Geometry check sheet. Reference: the model listing, model coordinates, mm. A direction names the side the tool comes from. Give positions to 0.01 mm unless a question says otherwise; leave off trailing zeros. Order: outer loops, then holes, each group sorted by start corner. A loop starts at its lowest first (then second) coordinate and runs counter-clockwise, first axis right, second up. Notation, with made-up numbers: M 63.5,36.25 L 81.5,36.25 A17 ccw 81.5,42.25 Z; hole C 43.25,40.25 d11. An arc over 180 degrees is marked long. Answer as CSV lines item,"result". Start each with the question number.
Q1. Set-up check for faces 5 (the flat face through (29, 0, 5)), 6 (the flat face through (118, 27, 5)), 7 (the flat face through (116, 33, 20)): record each of +Z, -Z, +X, -X, +Y, -Y from which the full face is reachable in a straight line by a thin tool's end or side.
Q2. Mould release check, pull along Y, two halves, no side actions. Record for faces 1 (the flat face through (30, 35, 5)), 2 (the cylindrical face through (77.51, 16.99, 19.65)), 3 (the cylindrical face through (140, 26, 20)), 4 (the flat face through (7, 25, 5)): +Y half, -Y half, draft (parallel to the pull), parting line (faces both ways), or undercut.
Q3. Section check D-D, the plane z = 37. Record the boundary of the cut face in (x, y).
Q4. Section check A-A, the plane z = 20. Record the boundary of the cut face in (x, y), then the cut area to 3 significant figures.
Q5. Go/stop test with flat-tipped pins: pin 1 (17.5 mm diameter, centred on x = 42, z = 29.5, fed in from -Y); pin 2 (7.5 mm diameter, centred on x = 11, z = 8.5, fed in from -Y); pin 3 (1 mm diameter, centred on x = 65, y = 27.5, fed in from -Z). Record where each tip stops, or that it passes through.
Q6. Section check C-C, the plane x = 51.5. Record the boundary of the cut face in (y, z), then the cut area to 3 significant figures.
Q7. Thickness scan on line 1 (Z direction, x = 125, y = 27.5); line 2 (X direction, y = 17.5, z = -3); line 3 (Y direction, x = 129, z = 7). Record the ranges inside material, lowest first.
Q8. Section check B-B, the plane x = 90. Record the boundary of the cut face in (y, z), then the cut area to 4 significant figures.
```python
from build123d import *

# Parameters (mm, degrees)
BOSS_EXTRUDE1_DEPTH       = 10
BOSS_EXTRUDE2_DEPTH       = 5
BOSS_EXTRUDE2_DEPTH_BACK  = 15
BOSS_EXTRUDE3_DEPTH       = 35
BOSS_EXTRUDE3_DEPTH_BACK  = 15
RIB27_REACH               = 125.11
SKETCH19_WALL_W           = 287.352003994
SKETCH19_WALL_H           = 10
BOSS_EXTRUDE4_DEPTH       = 5
RIB29_REACH               = 127.025
SKETCH20_WALL_W           = 301.546848684
SKETCH20_WALL_H           = 10
CUT_EXTRUDE1_START        = -5
CUT_EXTRUDE1_DEPTH        = 5
CUT_EXTRUDE2_DEPTH        = 5
SKETCH37_R                = 8
BOSS_EXTRUDE6_DEPTH       = 15.5
BOSS_EXTRUDE11_REACH      = 129.598
BOSS_EXTRUDE11_END_RADIUS = 22.5
SKETCH45_W                = 30
SKETCH45_H                = 15.5
BOSS_EXTRUDE12_START      = 5
BOSS_EXTRUDE12_DEPTH      = 30
SKETCH52_W                = 33.733601919
SKETCH52_H                = 5
CUT_EXTRUDE4_DEPTH        = 154.948043183


# Read off the part's stored shape, not the designer's step: Boss-Extrude12
with BuildPart() as part:
    # Sketch1 → Boss-Extrude1 (new body)
    with BuildSketch(Plane.XY):
        with BuildLine():
            Line((15, 0), (75.857864376, 0))
            ThreePointArc((75.857864376, 0), (67.5, 17.5), (75.857864376, 35))
            Line((75.857864376, 35), (15, 35))
            ThreePointArc((15, 35), (32.5, 17.5), (15, 0))
        make_face()
    extrude(amount=BOSS_EXTRUDE1_DEPTH)

    # Sketch2 → Boss-Extrude2 (add, two sides: drawn at the far end of the back side and taken through both)
    with BuildSketch(Plane.XY.offset(10).offset(-BOSS_EXTRUDE2_DEPTH_BACK)):
        with BuildLine():
            Line((15, 10), (0, 10))
            Line((0, 10), (0, 0))
            Line((0, 0), (15, 0))
            ThreePointArc((15, 0), (32.5, 17.5), (15, 35))
            Line((15, 35), (0, 35))
            Line((0, 35), (0, 25))
            Line((0, 25), (15, 25))
            ThreePointArc((15, 25), (22.5, 17.5), (15, 10))
        make_face()
    extrude(amount=BOSS_EXTRUDE2_DEPTH + BOSS_EXTRUDE2_DEPTH_BACK)

    # Sketch3 → Boss-Extrude3 (add, two sides: drawn at the far end of the back side and taken through both)
    with BuildSketch(Plane.XY.offset(10).offset(-BOSS_EXTRUDE3_DEPTH_BACK)):
        with BuildLine():
            Line((102.247448714, 20), (112.360679775, 20))
            ThreePointArc((112.360679775, 20), (67.5, 17.5), (112.360679775, 15))
            Line((112.360679775, 15), (102.247448714, 15))
            ThreePointArc((102.247448714, 15), (77.5, 17.5), (102.247448714, 20))
        make_face()
    extrude(amount=BOSS_EXTRUDE3_DEPTH + BOSS_EXTRUDE3_DEPTH_BACK)

    # Sketch19 wall → Rib27 (add, up to next)
    with BuildSketch(Plane(origin=(50, 17.5, 18.75), x_dir=(0.894427191, 0, 0.4472135955), z_dir=(0.4472135955, 0, -0.894427191)), mode=Mode.PRIVATE) as rib27_sk1:
        Rectangle(SKETCH19_WALL_W, SKETCH19_WALL_H)
    rib27_tool1 = extrude(rib27_sk1.sketch, amount=RIB27_REACH, mode=Mode.PRIVATE) - part.part
    add(rib27_tool1.solids().sort_by_distance((50, 17.5, 18.75))[0])

    # Sketch21 → Boss-Extrude4 (add)
    with BuildSketch(Plane.XY.offset(45)):
        with BuildLine():
            Line((102.247448714, 20), (112.360679775, 20))
            ThreePointArc((112.360679775, 20), (67.5, 17.5), (112.360679775, 15))
            Line((112.360679775, 15), (102.247448714, 15))
            ThreePointArc((102.247448714, 15), (77.5, 17.5), (102.247448714, 20))
        make_face()
    extrude(amount=BOSS_EXTRUDE4_DEPTH)

    # Sketch20 wall → Rib29 (add, up to next)
    with BuildSketch(Plane(origin=(50, 17.5, 27.5), x_dir=(0.707106781187, 0, 0.707106781187), z_dir=(0.707106781187, 0, -0.707106781187)), mode=Mode.PRIVATE) as rib29_sk1:
        Rectangle(SKETCH20_WALL_W, SKETCH20_WALL_H)
    rib29_tool1 = extrude(rib29_sk1.sketch, amount=RIB29_REACH, mode=Mode.PRIVATE) - part.part
    add(rib29_tool1.solids().sort_by_distance((50, 17.5, 27.5))[0])

    # Sketch23 → Cut-Extrude1 (cut)
    with BuildSketch(Plane.XY.offset(50).offset(CUT_EXTRUDE1_START)):
        with BuildLine():
            Line((102.247448714, 20), (112.360679775, 20))
            ThreePointArc((112.360679775, 20), (67.5, 17.5), (112.360679775, 15))
            Line((112.360679775, 15), (102.247448714, 15))
            ThreePointArc((102.247448714, 15), (77.5, 17.5), (102.247448714, 20))
        make_face()
    extrude(amount=CUT_EXTRUDE1_DEPTH, mode=Mode.SUBTRACT)

    # Sketch25 → Cut-Extrude2 (cut)
    with BuildSketch(Plane.ZY.offset(-67.5)):
        Polygon((45, 17.5), (45, 9.449706044), (52.526454381, 9.449706044), (52.526454381, 28.660137354), (45, 28.660137354), align=None)
    extrude(amount=-CUT_EXTRUDE2_DEPTH, mode=Mode.SUBTRACT)



with BuildPart() as body_2:
    # Sketch37 → Boss-Extrude6 (new, symmetric)
    with BuildSketch(Plane(origin=(0, 17.5, 0), x_dir=(-1, 0, 0), z_dir=(0, -1, 0))):
        with BuildLine():
            Line((-125, -5), (-112.5, -5))
            Line((-112.5, -5), (-112.5, -35))
            Line((-112.5, -35), (-125, -35))
            ThreePointArc((-125, -35), (-140, -20), (-125, -5))
        make_face()
        with Locations(Location((-125, -20, 0), (0, 0, 90))):
            Circle(SKETCH37_R, mode=Mode.SUBTRACT)
    extrude(amount=BOSS_EXTRUDE6_DEPTH, both=True)


with BuildPart() as part_1:
    add(part.part)

    add(body_2.part)  # Boss-Extrude11 merges body 2
    # Boss-Extrude11: up to this cylinder (the profile starts outside it)
    boss_extrude11_end = Plane(origin=(90, 17.5, 20), z_dir=(0, 0, 1)) * Cylinder(BOSS_EXTRUDE11_END_RADIUS, 305.196, mode=Mode.PRIVATE)
    # Sketch45 → Boss-Extrude11 (add, up to the surface)
    with BuildSketch(Plane.ZY.offset(-112.5), mode=Mode.PRIVATE) as boss_extrude11_sk1:
        with Locations((20, 9.75)):
            Rectangle(SKETCH45_W, SKETCH45_H)
    boss_extrude11_tool1 = extrude(boss_extrude11_sk1.sketch, amount=BOSS_EXTRUDE11_REACH, mode=Mode.PRIVATE) - boss_extrude11_end
    add(boss_extrude11_tool1.solids().sort_by_distance((112.5, 9.75, 20))[0])

    # Boss-Extrude12 outline → Boss-Extrude12 (add)
    with BuildSketch(Plane.XY.offset(BOSS_EXTRUDE12_START)):
        with BuildLine():
            ThreePointArc((112.360679775, 20), (112.465142943, 18.751939508), (112.5, 17.5))
            Line((112.5, 17.5), (112.5, 33))
            Line((112.5, 33), (106.30950643, 33))
            ThreePointArc((106.30950643, 33), (110.39842703, 26.994955224), (112.360679775, 20))
        make_face()
    extrude(amount=BOSS_EXTRUDE12_DEPTH)

    # Sketch52 → Cut-Extrude4 (cut, through all)
    with BuildSketch(Plane.XY.offset(45)):
        with Locations((129.227480735, 17.5)):
            Rectangle(SKETCH52_W, SKETCH52_H)
    extrude(amount=-CUT_EXTRUDE4_DEPTH, mode=Mode.SUBTRACT)


solid = part_1.part
```
Answer block:
1,face 5,"+Z, -Z, -X, -Y"
1,face 6,"-Z, +X, +Y"
1,face 7,"+Z, -Z, +X, +Y"
2,face 1,"+Y half"
2,face 2,"undercut"
2,face 3,"draft"
2,face 4,"undercut"
3,outline,"M 59.5,12.5 L 68.06,12.5 A22.5 ccw 112.36,15 L 102.25,15 A12.5 cw long 102.25,20 L 112.36,20 A22.5 ccw 68.06,22.5 L 59.5,22.5 Z"
4,outline,"M 42.5,12.5 L 68.06,12.5 A22.5 ccw 106.31,2 L 117,2 L 117,15 L 102.25,15 A12.5 cw long 102.25,20 L 117,20 L 117,33 L 106.31,33 A22.5 ccw 68.06,22.5 L 42.5,22.5 Z; M 133,2 L 140,2 L 140,15 L 133,15 Z; M 133,20 L 140,20 L 140,33 L 133,33 Z"
4,area,"1,660 mm2"
5,pin 1,"stops at y = 12.5"
5,pin 2,"stops at y = 0"
5,pin 3,"stops at z = 0"
6,outline,"M 0,0 L 35,0 L 35,10 L 22.5,10 L 22.5,29 L 12.5,29 L 12.5,10 L 0,10 Z"
6,area,"540 mm2"
7,line 1,"z = 5 to 12, 28 to 35"
7,line 2,"x = 22.5 to 32.5, 67.5 to 77.5"
7,line 3,"y = 2 to 15, 20 to 33"
8,outline,"M -5,-5 L 5,-5 L 5,45 L -5,45 Z; M 30,-5 L 40,-5 L 40,45 L 30,45 Z"
8,area,"1,000 mm2"
